```python
from build123d import *

# Parameters (mm, degrees)
SKETCH1_W           = 50
SKETCH1_H           = 120
SKETCH1_R           = 2.1
SKETCH1_R_2         = 1.6
BOSS_EXTRUDE1_DEPTH = 5
FILLET2_R           = 5


with BuildPart() as part:
    # Sketch1 → Boss-Extrude1 (new body)
    with BuildSketch(Plane(origin=(0, 0, 0), x_dir=(1, 0, 0), z_dir=(0, 1, 0))):
        Rectangle(SKETCH1_W, SKETCH1_H)
        with Locations((-15, 50)):
            Circle(SKETCH1_R, mode=Mode.SUBTRACT)
        with Locations((15, 50)):
            Circle(SKETCH1_R, mode=Mode.SUBTRACT)
        with Locations((15, 22.5)):
            Circle(SKETCH1_R_2, mode=Mode.SUBTRACT)
        with Locations((-15, -27.5)):
            Circle(SKETCH1_R_2, mode=Mode.SUBTRACT)
        with Locations((-15, -17.5)):
            Circle(SKETCH1_R_2, mode=Mode.SUBTRACT)
        with Locations((-15, -7.5)):
            Circle(SKETCH1_R_2, mode=Mode.SUBTRACT)
        with Locations((15, -27.5)):
            Circle(SKETCH1_R_2, mode=Mode.SUBTRACT)
        with Locations((15, -17.5)):
            Circle(SKETCH1_R_2, mode=Mode.SUBTRACT)
        with Locations((15, -7.5)):
            Circle(SKETCH1_R_2, mode=Mode.SUBTRACT)
        with Locations((-15, 2.5)):
            Circle(SKETCH1_R_2, mode=Mode.SUBTRACT)
        with Locations((-15, 12.5)):
            Circle(SKETCH1_R_2, mode=Mode.SUBTRACT)
        with Locations((-15, 22.5)):
            Circle(SKETCH1_R_2, mode=Mode.SUBTRACT)
        with Locations((15, 2.5)):
            Circle(SKETCH1_R_2, mode=Mode.SUBTRACT)
        with Locations((15, 12.5)):
            Circle(SKETCH1_R_2, mode=Mode.SUBTRACT)
        with Locations((15, -50)):
            Circle(SKETCH1_R, mode=Mode.SUBTRACT)
        with Locations((-15, -50)):
            Circle(SKETCH1_R, mode=Mode.SUBTRACT)
    extrude(amount=BOSS_EXTRUDE1_DEPTH)

    # Fillet2
    fillet2_edges = [part.edges().sort_by_distance(p)[0] for p in [
        (25, 2.5, 60),
        (-25, 2.5, 60),
        (-25, 2.5, -60),
        (25, 2.5, -60),
    ]]
    fillet(fillet2_edges, radius=FILLET2_R)


solid = part.part
```
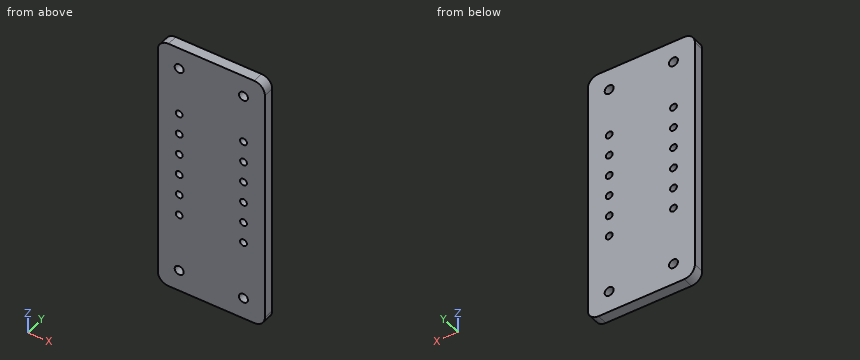
Source: CAD feature listing. Evaluate the final solid. Frame: model axes, mm. Coordinates: 2 decimals unless noted, no trailing zeros. Write each loop counter-clockwise with the first axis right and the second up, starting at its lowest first coordinate (ties: lowest second). Pieces come first, ordered by that corner, then holes. Notation, with made-up numbers: (60, -35.5) - (90, -35.5) arc R22 cw to (90, -1.5) - close; hole circle Ø4 at (49.5, -15.75). An arc over 180 degrees is marked (long way). Answer as a JSON object with one key per item and string values.
Q1. Material intervals for line 1 (X direction, y = 2.55, z = -2.5); line 2 (X direction, y = 1.65, z = -50); line 3 (Z direction, x = 21, y = 1.65), sorted ascending. Write a range as [from, to].
Ans:
{"line 1": "x = [-25, -16.6], [-13.4, 13.4], [16.6, 25]", "line 2": "x = [-25, -17.1], [-12.9, 12.9], [17.1, 25]", "line 3": "z = [-59.9, 59.9]"}
Q2. Section query B-B, the plane y = 0.75. State how many separate pieces and enclosed holes the cut face has, plus the area to 3 significant figures.
Ans:
{"separate pieces": "1", "enclosed holes": "16", "area": "5,830 mm2"}
Q3. Section query A-A, the plane z = -2.5. Output: boundary loops of the cut face in (x, y), plus the area to 3 significant figures.
Ans:
{"outline": "(-25, 0) - (-16.6, 0) - (-16.6, 5) - (-25, 5) - close; (-13.4, 0) - (13.4, 0) - (13.4, 5) - (-13.4, 5) - close; (16.6, 0) - (25, 0) - (25, 5) - (16.6, 5) - close", "area": "218 mm2"}
